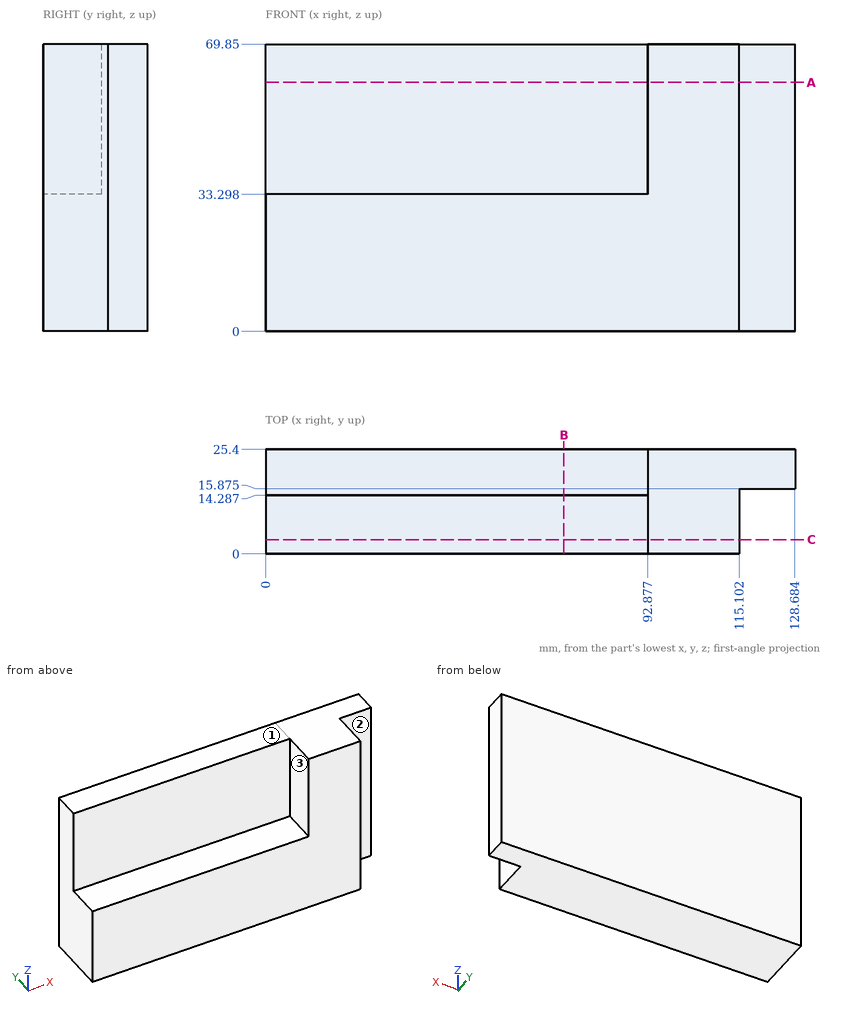
Could you check a few things on this drawing? It's one solid part, dimensions in mm from its lowest x, y, z. A direction names the side the tool comes from. Give positions to 0.01 mm unless a question says otherwise; leave off trailing zeros. Write each loop counter-clockwise with the first axis right and the second up, starting at its lowest first coordinate (ties: lowest second). Pieces come first, ordered by that corner, then holes.
(1) If I drill on L1, parallel to X at y = 11.5, z = 45.5; L2, parallel to X at y = 1.5, z = 20; L3, parallel to Z at x = 77.5, y = 2.5, over which ranges is the centre line in solid material (lowest first)?
Output values:
L1: x = 92.88 to 115.1
L2: x = 0 to 115.1
L3: z = 0 to 33.3
(2) On a 3-axis mill with a long thin cutter (end or side, diameter ignored), from which of +Z, -Z, +X, -X, +Y, -Y can I reach the whole of each face in a straight line? I mean the marked faces 1, 2 and 3. Say none if no direction works.
Output values:
face 1: +Z, +X, -X, +Y, -Y
face 2: +Z, -Z, +X, -Y
face 3: +Z, -X, -Y
(3) Will these pins go through, and if not, where does the flat tip stop? pin 1 (7 mm diameter, centred on x = 54, y = 10, fed in from +Z); pin 2 (8 mm diameter, centred on y = 8.5, z = 19.5, fed in from +X); pin 3 (7 mm diameter, centred on x = 121, z = 19, fed in from -Y) (1 decimal).
Output values:
pin 1: stops at z = 33.3
pin 2: stops at x = 115.1
pin 3: stops at y = 15.9
(4) Imagine slicing it at B-B, the plane x = 72.5. Write out the boundary of the cut face in (y, z).
Output values:
outline: (0, 0) - (25.4, 0) - (25.4, 69.85) - (14.29, 69.85) - (14.29, 33.3) - (0, 33.3) - close
(5) Imagine slicing it at C-C, the plane y = 3.5. Write out the boundary of the cut face in (x, z), and give its area (4 significant figures).
Output values:
outline: (0, 0) - (115.1, 0) - (115.1, 69.85) - (92.88, 69.85) - (92.88, 33.3) - (0, 33.3) - close
area: 4,645 mm2
(6) Imagine slicing it at A-A, the plane z = 60.5. Write out the boundary of the cut face in (x, y) (1 decimal), and give its area (3 significant figures).
Output values:
outline: (0, 14.3) - (92.9, 14.3) - (92.9, 0) - (115.1, 0) - (115.1, 15.9) - (128.7, 15.9) - (128.7, 25.4) - (0, 25.4) - close
area: 1,730 mm2
